```python
from build123d import *

# Parameters (mm, degrees)
CROQUIS1_W                       = 10
CROQUIS1_H                       = 6
CROQUIS1_W_2                     = 4
CROQUIS1_H_2                     = 140
CROQUIS1_W_3                     = 6
SALIENTE_EXTRUIR1_DEPTH          = 6
TALADRO_DE_MARGEN_PARA_M31_D     = 3.6
TALADRO_DE_MARGEN_PARA_M31_DEPTH = 3
TALADRO_DE_MARGEN_PARA_M31_TIP   = 1.081549114
TALADRO_DE_MARGEN_PARA_M32_D     = 3.6
TALADRO_DE_MARGEN_PARA_M32_DEPTH = 8.6
TALADRO_DE_MARGEN_PARA_M32_TIP   = 1.081549114


with BuildPart() as part:
    # Croquis1 → Saliente-Extruir1 (new body)
    with BuildSketch(Plane.XY):
        with Locations((9, 137)):
            Rectangle(CROQUIS1_W, CROQUIS1_H)
        with Locations((2, 70)):
            Rectangle(CROQUIS1_W_2, CROQUIS1_H_2)
        with Locations((7, 3)):
            Rectangle(CROQUIS1_W_3, CROQUIS1_H)
    extrude(amount=SALIENTE_EXTRUIR1_DEPTH)

    # Taladro de margen para M31
    with Locations(Plane(origin=(14, 0, 0), x_dir=(0, 0, -1), z_dir=(1, 0, 0))):
        with Locations((-3, 137)):
            Hole(TALADRO_DE_MARGEN_PARA_M31_D / 2, depth=TALADRO_DE_MARGEN_PARA_M31_DEPTH)
            with Locations((0, 0, -(TALADRO_DE_MARGEN_PARA_M31_DEPTH + TALADRO_DE_MARGEN_PARA_M31_TIP / 2))):  # 118° drill point
                Cone(0, TALADRO_DE_MARGEN_PARA_M31_D / 2, TALADRO_DE_MARGEN_PARA_M31_TIP, mode=Mode.SUBTRACT)

    # Taladro de margen para M32
    with Locations(Plane(origin=(10, 0, 0), x_dir=(0, 0, -1), z_dir=(1, 0, 0))):
        with Locations((-3, 3)):
            Hole(TALADRO_DE_MARGEN_PARA_M32_D / 2, depth=TALADRO_DE_MARGEN_PARA_M32_DEPTH)
            with Locations((0, 0, -(TALADRO_DE_MARGEN_PARA_M32_DEPTH + TALADRO_DE_MARGEN_PARA_M32_TIP / 2))):  # 118° drill point
                Cone(0, TALADRO_DE_MARGEN_PARA_M32_D / 2, TALADRO_DE_MARGEN_PARA_M32_TIP, mode=Mode.SUBTRACT)


solid = part.part
```
Geometry: final body of the model. Coordinates: model frame, mm. A direction names the side the tool comes from. Round coordinates to 2 decimals unless told otherwise and drop trailing zeros. Loops run counter-clockwise (first coordinate to the right, second up) from the corner with the lowest first, then second, coordinate; pieces in that order, holes last. Notation, with made-up numbers: (-19.5, 84.25) -> (11.5, 84.25) arc R15 cw to (11.5, 100.25) -> close; hole circle Ø9 at (-26, 68.5). An arc over 180 degrees is marked (long way). Use one line per item in the form item = value.
Item 1: Contact query for flat-ended pins moving along their axis: pin 1 Ø2 at (y, z) = (112, 1.5) entering from -X; pin 2 Ø1 at (y, z) = (17, 5) entering from +X. Output: stop coordinate, or through.
Evaluation:
pin_1 = 0
pin_2 = 4
Item 2: Access query for faces 4 (the flat face through (10, 1.6, 1.6)), 5 (the cylindrical face through (5.64, 4.518, 3.968)), 6 (the flat face through (9, 134, 3)). Directions: +Z, -Z, +X, -X, +Y, -Y. A direction counts if a zero-diameter tool reaches every point of the face in a straight line with its end or side. Return the directions, or none.
Evaluation:
face_4 = +Z, -Z, +X, -Y
face_5 = +X
face_6 = +Z, -Z, +X
Item 3: Material intervals for probe 1 along Y at (x, z) = (5, 3.15); probe 2 along Y at (x, z) = (7, 0.5); probe 3 along Y at (x, z) = (8.25, 3.75), sorted ascending.
Evaluation:
probe_1 = 0 to 1.21, 4.79 to 6, 134 to 140
probe_2 = 0 to 6, 134 to 140
probe_3 = 0 to 1.36, 4.64 to 6, 134 to 140
Item 4: Cut plane B-B on y = 54.5. Output: boundary loops of the cut face in (x, z).
Evaluation:
outline = (0, 0) -> (4, 0) -> (4, 6) -> (0, 6) -> close
Item 5: Cut plane A-A on x = 8. Output: boundary loops of the cut face in (y, z).
Evaluation:
outline = (0, 0) -> (6, 0) -> (6, 6) -> (0, 6) -> close; (134, 0) -> (140, 0) -> (140, 6) -> (134, 6) -> close; hole circle Ø3.6 at (3, 3)
Item 6: Draft query along Y for faces 1 (the flat face through (4, 69, 3)), 2 (the flat face through (0, 69, 3)), 3 (the flat face through (5, 0, 3)). Return one class per face: released by +Y, released by -Y, zero draft, split by the parting line, or undercut.
Evaluation:
face_1 = undercut
face_2 = zero draft
face_3 = released by -Y
